Design review of the part built by this model. Coordinates are the model's own, in mm. A direction names the side the tool comes from. Coordinates: 2 decimals unless noted, no trailing zeros. Write each loop counter-clockwise with the first axis right and the second up, starting at its lowest first coordinate (ties: lowest second). Pieces come first, ordered by that corner, then holes.
Q1. For L1, parallel to Y at x = 0, z = 2.6; L2, parallel to Y at x = -14.5, z = -36; L3, parallel to X at y = 19, z = 2.5, list the stretches that pass through material, from the lowest coordinate up.
Q2. Take a section at B-B, the plane x = 0. Write out the cut boundary in (y, z) (3 decimals), plus the area to 3 significant figures.
Q3. Take a section at D-D, the plane y = 0. Write out the cut boundary in (x, z) (3 decimals).
Q4. For pin 1 Ø2.5 at (x, y) = (32, -51.5) entering from +Z (3 decimals); pin 2 Ø9 at (x, z) = (29.5, -7) entering from +Y; pin 3 Ø7 at (x, y) = (-17.02, -18.32) entering from -Z; pin 4 Ø10 at (x, z) = (17, -10.5) entering from -Y, all flat-tipped, find the tip position at first contact; note any pin that passes through.
Q5. The part is to be moulded in two halves that separate along Y. For faces 1 (the cylindrical face through (0.899, -83.465, 2.305)), 2 (the flat face through (32, 13.25, -11)), 3 (the cylindrical face through (18.72, -19.67, 2.54)), say which applies: released by +Y, released by -Y, zero draft, split by the parting line, or undercut.
Q6. Take a section at C-C, the plane z = -1.5. Write out the cut boundary in (x, y).
Q7. Take a section at A-A, the plane y = -63. Write out the cut boundary in (x, z) (3 decimals).
Q8. For faces 4 (the flat face through (-20, -81, -11)), 5 (the flat face through (29, -33, -12)), 6 (the cylindrical face through (-19.874, -83.535, 0.04)), 7 (the flat face through (-20, 7, 5)), 8 (the cylindrical face through (31.535, -3.376, -18.191)), list the 3-axis set-ups (+Z, -Z, +X, -X, +Y, -Y) from which the entire face can be reached by the end or side of a thin tool; tool diameter is ignored.
from build123d import *

# Parameters (mm, degrees)
SKETCH1_R           = 20.45
BOSS_EXTRUDE2_DEPTH = 5
BOSS_EXTRUDE3_DEPTH = 5
SKETCH14_R          = 20.45
BOSS_EXTRUDE6_DEPTH = 5
CUT_EXTRUDE2_DEPTH  = 5
BOSS_EXTRUDE7_DEPTH = 26.5
BOSS_EXTRUDE8_DEPTH = 26.5
CUT_EXTRUDE3_DEPTH  = 26.5
SKETCH24_R          = 2.25
CUT_EXTRUDE5_DEPTH  = 10
SKETCH25_R          = 2.25
CUT_EXTRUDE6_DEPTH  = 10


with BuildPart() as part:
    # Sketch1 → Boss-Extrude2 (new body)
    with BuildSketch(Plane.XY):
        with BuildLine():
            Line((29, 13.25), (25.796075283, 13.25))
            ThreePointArc((25.796075283, 13.25), (-29, 0), (25.796075283, -13.25))
            Line((25.796075283, -13.25), (29, -13.25))
            Line((29, -13.25), (29, 13.25))
        make_face()
        Circle(SKETCH1_R, mode=Mode.SUBTRACT)
    extrude(amount=BOSS_EXTRUDE2_DEPTH)



with BuildPart() as body_2:
    # Sketch2 → Boss-Extrude3 (new body)
    with BuildSketch(Plane(origin=(29, 0, 0), x_dir=(0, 0, -1), z_dir=(1, 0, 0))):
        with BuildLine():
            Line((0, 13.25), (26.375, 13.25))
            ThreePointArc((26.375, 13.25), (29.910533906, 11.785533906), (31.375, 8.25))
            Line((31.375, 8.25), (31.375, -81))
            Line((31.375, -81), (0, -81))
            Line((0, -81), (0, -13.25))
            Line((0, -13.25), (0, 13.25))
        make_face()
    extrude(amount=BOSS_EXTRUDE3_DEPTH)

    # Sketch17 → Cut-Extrude2 (cut)
    with BuildSketch(Plane(origin=(34, 0, 0), x_dir=(0, 0, -1), z_dir=(1, 0, 0))):
        with BuildLine():
            Line((0, -13.25), (3.875, -13.25))
            ThreePointArc((3.875, -13.25), (4.582106781, -13.542893219), (4.875, -14.25))
            Line((4.875, -14.25), (4.875, -81))
            Line((4.875, -81), (0, -81))
            Line((0, -81), (0, -13.25))
        make_face()
    extrude(amount=-CUT_EXTRUDE2_DEPTH, mode=Mode.SUBTRACT)


with BuildPart() as body_3:
    # Sketch14 → Boss-Extrude6 (new body)
    with BuildSketch(Plane.XZ.offset(81)):
        with BuildLine():
            Line((29, -4.875), (25.796075283, -4.875))
            ThreePointArc((25.796075283, -4.875), (-29, -18.125), (25.796075283, -31.375))
            Line((25.796075283, -31.375), (29, -31.375))
            Line((29, -31.375), (29, -4.875))
        make_face()
        with Locations(Location((0, -18.125, 0), (0, 0, 270))):
            Circle(SKETCH14_R, mode=Mode.SUBTRACT)
    extrude(amount=BOSS_EXTRUDE6_DEPTH)


with BuildPart() as part_1:
    add(part.part)

    add(body_2.part)  # Boss-Extrude7 merges body 2
    # Sketch21 → Boss-Extrude7 (add)
    with BuildSketch(Plane(origin=(0, 13.25, 0), x_dir=(1, 0, 0), z_dir=(0, 1, 0))):
        with BuildLine():
            Line((29, 0), (29, -5))
            ThreePointArc((29, -5), (32.535533906, -3.535533906), (34, 0))
            Line((34, 0), (29, 0))
        make_face()
    extrude(amount=-BOSS_EXTRUDE7_DEPTH)


    add(body_3.part)  # Boss-Extrude8 merges body 3
    # Sketch22 → Boss-Extrude8 (add)
    with BuildSketch(Plane.XY.offset(-4.875)):
        with BuildLine():
            ThreePointArc((29, -86), (32.535533906, -84.535533906), (34, -81))
            Line((34, -81), (29, -81))
            Line((29, -81), (29, -86))
        make_face()
    extrude(amount=-BOSS_EXTRUDE8_DEPTH)

    # Sketch23 → Cut-Extrude3 (cut)
    with BuildSketch(Plane(origin=(34, 0, 0), x_dir=(0, 0, -1), z_dir=(1, 0, 0))):
        with BuildLine():
            Line((15.125, -6.375), (15.125, -36.375))
            Line((15.125, -36.375), (18.125, -36.375))
            Line((18.125, -36.375), (21.125, -36.375))
            Line((21.125, -36.375), (21.125, -6.375))
            ThreePointArc((21.125, -6.375), (18.125, -3.375), (15.125, -6.375))
        make_face()
        with BuildLine():
            Line((21.125, -36.375), (18.125, -36.375))
            Line((18.125, -36.375), (18.125, -69.375))
            ThreePointArc((18.125, -69.375), (20.246320344, -68.496320344), (21.125, -66.375))
            Line((21.125, -66.375), (21.125, -36.375))
        make_face()
        with BuildLine():
            Line((18.125, -36.375), (15.125, -36.375))
            Line((15.125, -36.375), (15.125, -66.375))
            ThreePointArc((15.125, -66.375), (16.003679656, -68.496320344), (18.125, -69.375))
            Line((18.125, -69.375), (18.125, -36.375))
        make_face()
    extrude(amount=-CUT_EXTRUDE3_DEPTH, mode=Mode.SUBTRACT)

    # Sketch24 → Cut-Extrude5 (cut)
    with BuildSketch(Plane.XY.offset(5)):
        with Locations((17.67766953, 17.67766953)):
            Circle(SKETCH24_R)
        with Locations((17.67766953, -17.67766953)):
            Circle(SKETCH24_R)
        with Locations((-17.67766953, 17.67766953)):
            Circle(SKETCH24_R)
        with Locations((-17.01531967, -18.316083002)):
            Circle(SKETCH24_R)
    extrude(amount=-CUT_EXTRUDE5_DEPTH, mode=Mode.SUBTRACT)

    # Sketch25 → Cut-Extrude6 (cut)
    with BuildSketch(Plane.XZ.offset(86)):
        with Locations(Location((-17.67766953, -0.44733047, 0), (0, 0, 270))):
            Circle(SKETCH25_R)
        with Locations(Location((17.67766953, -0.44733047, 0), (0, 0, 270))):
            Circle(SKETCH25_R)
        with Locations(Location((17.67766953, -35.80266953, 0), (0, 0, 270))):
            Circle(SKETCH25_R)
        with Locations(Location((-17.67766953, -35.80266953, 0), (0, 0, 270))):
            Circle(SKETCH25_R)
    extrude(amount=-CUT_EXTRUDE6_DEPTH, mode=Mode.SUBTRACT)


solid = part_1.part
Responses:
1. L1: y = -86 to -81, -29 to -20.45, 20.45 to 29
1. L2: y = -86 to -81
1. L3: x = -21.91 to -19.5, -15.86 to -7.56, 7.56 to 15.86, 19.5 to 21.91
2. outline: (-86, -47.125) - (-81, -47.125) - (-81, -38.575) - (-86, -38.575) - close; (-86, 2.325) - (-81, 2.325) - (-81, 10.875) - (-86, 10.875) - close; (-29, 0) - (-20.45, 0) - (-20.45, 5) - (-29, 5) - close; (20.45, 0) - (29, 0) - (29, 5) - (20.45, 5) - close
2. area: 171 mm2
3. outline: (-29, 0) - (-20.45, 0) - (-20.45, 5) - (-29, 5) - close; (20.45, 0) - (29, 0) - (29, -31.375) - (34, -31.375) - (34, 0) arc R5 ccw to (29, 5) - (20.45, 5) - close
4. pin 1: stops at z = -4.875
4. pin 2: stops at y = 13.25
4. pin 3: stops at z = 0
4. pin 4: stops at y = -86
5. face 1: zero draft
5. face 2: released by +Y
5. face 3: undercut
6. outline: (-23.76, -86) - (-19.67, -86) - (-19.67, -81) - (-23.76, -81) - close; (-15.69, -86) - (-11.91, -86) - (-11.91, -81) - (-15.69, -81) - close; (11.91, -86) - (15.69, -86) - (15.69, -81) - (11.91, -81) - close; (19.67, -86) - (23.76, -86) - (23.76, -81) - (19.67, -81) - close; (29, -13.25) - (34, -13.25) - (34, 13.25) - (29, 13.25) - close
7. outline: (29, -31.375) - (34, -31.375) - (34, -21.125) - (29, -21.125) - close; (29, -15.125) - (34, -15.125) - (34, -4.875) - (29, -4.875) - close
8. face 4: +Z, -Z, -X
8. face 5: -Z, -X, +Y
8. face 6: -Y
8. face 7: +Z, +X, -X, +Y
8. face 8: +X, -X
